Here's how the part is built. I have some questions about the finished solid (model axes, mm). Face numbers are marked on the shaded views. A direction names the side the tool comes from. Round coordinates to 2 decimals unless told otherwise and drop trailing zeros. Order: outer loops, then holes, each group sorted by start corner. A loop starts at its lowest first (then second) coordinate and runs counter-clockwise, first axis right, second up.
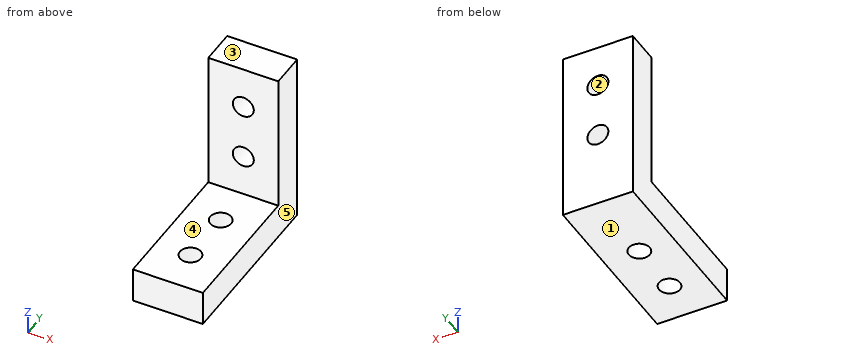
```python
from build123d import *

# Parameters (mm, degrees)
SKETCH_W     = 10
SKETCH_H     = 25
SKETCH_R     = 1.5
PAD_DEPTH    = 5
SKETCH001_W  = 10
SKETCH001_H  = 5
PAD001_DEPTH = 20
SKETCH002_R  = 1.5
POCKET_DEPTH = 25.001


with BuildPart() as part:
    # Sketch → Pad (new body)
    with BuildSketch(Plane.XY):
        with Locations((5, 12.5)):
            Rectangle(SKETCH_W, SKETCH_H)
        with Locations((5, 14)):
            Circle(SKETCH_R, mode=Mode.SUBTRACT)
        with Locations((5, 6)):
            Circle(SKETCH_R, mode=Mode.SUBTRACT)
    extrude(amount=PAD_DEPTH)

    # Sketch001 → Pad001 (new body)
    with BuildSketch(Plane.XY.offset(5)):
        with Locations((5, 22.5)):
            Rectangle(SKETCH001_W, SKETCH001_H)
    extrude(amount=PAD001_DEPTH)

    # Sketch002 → Pocket (cut, through all)
    with BuildSketch(Plane(origin=(0, 25, 0), x_dir=(-1, 0, 0), z_dir=(0, 1, 0))):
        with Locations((-5, 19)):
            Circle(SKETCH002_R)
        with Locations((-5, 11)):
            Circle(SKETCH002_R)
    extrude(amount=-POCKET_DEPTH, mode=Mode.SUBTRACT)


solid = part.part
```
1) We'd pull the mould along Z, two halves only. Please class the marked faces 1, 2 and 3: +Z half, -Z half, draft (parallel to the pull), parting line (faces both ways), or undercut.
2) For the marked faces 4 and 5, which set-ups out of +Z, -Z, +X, -X, +Y, -Y let a thin tool reach every point of the face, with its end or its side?
3) If we section it at A-A (x = 5): Write out the boundary of the cut face in (y, z).
4) I need wall thicknesses on line 1 (Z direction, x = 5, y = 22); line 2 (Y direction, x = 4.25, z = 5.25); line 3 (Z direction, x = 9.25, y = 18.5). Which ranges of each line are inside material? Lowest first, please.
5) I'm going to push flat-ended pins straight in: pin 1 (3.5 mm diameter, centred on x = 5, y = 14, fed in from -Z); pin 2 (3 mm diameter, centred on x = 4, z = 12.5, fed in from -Y); pin 3 (2 mm diameter, centred on x = 8, y = 4.5, fed in from +Z). Where does each tip first touch, or does it pass through?
6) If we section it at B-B (z = 19): Write out the boundary of the cut face in (x, y).
7) If we section it at D-D (z = 4.25): Write out the boundary of the cut face in (x, y).
8) If we section it at C-C (y = 6): Write out the boundary of the cut face in (x, z).
Solutions:
1. face 1: -Z half
1. face 2: undercut
1. face 3: +Z half
2. face 4: +Z, +X, -X, -Y
2. face 5: +Z, -Z, +X, +Y, -Y
3. outline: (0, 0) - (4.5, 0) - (4.5, 5) - (0, 5) - close; (7.5, 0) - (12.5, 0) - (12.5, 5) - (7.5, 5) - close; (15.5, 0) - (25, 0) - (25, 9.5) - (20, 9.5) - (20, 5) - (15.5, 5) - close; (20, 12.5) - (25, 12.5) - (25, 17.5) - (20, 17.5) - close; (20, 20.5) - (25, 20.5) - (25, 25) - (20, 25) - close
4. line 1: z = 0 to 9.5, 12.5 to 17.5, 20.5 to 25
4. line 2: y = 20 to 25
4. line 3: z = 0 to 5
5. pin 1: stops at z = 0
5. pin 2: stops at y = 20
5. pin 3: stops at z = 5
6. outline: (0, 20) - (3.5, 20) - (3.5, 25) - (0, 25) - close; (6.5, 20) - (10, 20) - (10, 25) - (6.5, 25) - close
7. outline: (0, 0) - (10, 0) - (10, 25) - (0, 25) - close; hole circle Ø3 at (5, 6); hole circle Ø3 at (5, 14)
8. outline: (0, 0) - (3.5, 0) - (3.5, 5) - (0, 5) - close; (6.5, 0) - (10, 0) - (10, 5) - (6.5, 5) - close
